Read the model definition and answer for the solid it produces. Units are mm, in the model's axes. A direction names the side the tool comes from. Coordinates: 2 decimals unless noted, no trailing zeros. Order: outer loops, then holes, each group sorted by start corner. A loop starts at its lowest first (then second) coordinate and runs counter-clockwise, first axis right, second up. Notation, with made-up numbers: (-39.5, -5) -> (-25.5, -5) arc R25 cw to (-25.5, 29) -> close; hole circle Ø6 at (33, 88.25). An arc over 180 degrees is marked (long way). Use CSV: the item, a comma, the result in double quotes.
```python
from build123d import *

# Parameters (mm, degrees)
F1_DEPTH    = 8
F3_DEPTH    = 12
F4_R        = 1.5
F5_R        = 1.5
F6_T1_DEPTH = 118.05


# Not quite as in the source:
# - a fillet or chamfer that OpenCascade refuses, or shapes differently, is made with other operations: its cross-section is extruded or revolved along the edge and cut away or added


with BuildPart() as f1:
    # F0 (on Top) → F1 (new body)
    with BuildSketch(Plane.XY):
        Polygon((-127.8, 0), (-132.3, 0), (-132.3, -29), (-129.3, -29), (-129.3, -91.6), (3.75, -91.6), (3.75, -29), (6.75, -29), (6.75, 0), (2.25, 0), (2.25, -20), (-2.25, -20), (-2.25, 0), (-6.75, 0), (-6.75, -29), (-3.75, -29), (-3.75, -84.1), (-121.8, -84.1), (-121.8, -29), (-118.8, -29), (-118.8, 0), (-123.3, 0), (-123.3, -20), (-127.8, -20), align=None)
    extrude(amount=F1_DEPTH)

    # F2 (on face) → F3 (join)
    with BuildSketch(Plane.XY.offset(8)):
        Polygon((-127.8, 0), (-132.3, 0), (-132.3, -29), (-118.8, -29), (-118.8, 0), (-123.3, 0), (-123.3, -20), (-127.8, -20), align=None)
        Polygon((-2.25, 0), (-6.75, 0), (-6.75, -29), (6.75, -29), (6.75, 0), (2.25, 0), (2.25, -20), (-2.25, -20), align=None)
    extrude(amount=F3_DEPTH)

    # F4
    f4_edges = [f1.edges().sort_by_distance(p)[0] for p in [
        (-129.3, -29, 4),
        (-125.55, -29, 8),
        (-121.8, -29, 4),
        (-3.75, -29, 4),
        (0, -29, 8),
        (3.75, -29, 4),
    ]]
    fillet(f4_edges, radius=F4_R)

    # F5
    f5_edges = [f1.edges().sort_by_distance(p)[0] for p in [
        (-132.3, -29, 10),
        (-125.55, -29, 20),
        (-118.8, -29, 10),
        (6.75, -29, 10),
        (0, -29, 20),
        (-6.75, -29, 10),
    ]]
    fillet(f5_edges, radius=F5_R)

    # F6: fillet of radius 5 on 2 edges, made by hand

    # F6_s2 → F6_t1 (cut)
    with BuildSketch(Plane.YZ.offset(-121.8)):
        with BuildLine():
            ThreePointArc((-84.1, 3), (-85.5644660941, 6.5355339059), (-89.1, 8))
            Line((-89.1, 8), (-84.1, 8))
            Line((-84.1, 8), (-84.1, 3))
        make_face()
        with BuildLine():
            ThreePointArc((-89.1, 0), (-85.5644660941, 1.4644660941), (-84.1, 5))
            Line((-84.1, 5), (-84.1, 0))
            Line((-84.1, 0), (-89.1, 0))
        make_face()
    extrude(amount=F6_T1_DEPTH, mode=Mode.SUBTRACT)


solid = f1.part
```
Item 1: Find section B-B, the plane z = 16. Give the vertices of the cut face in (x, y).
Return value:
outline,"(-132.3, -27.5) arc R1.5 ccw to (-130.8, -29) -> (-120.3, -29) arc R1.5 ccw to (-118.8, -27.5) -> (-118.8, 0) -> (-123.3, 0) -> (-123.3, -20) -> (-127.8, -20) -> (-127.8, 0) -> (-132.3, 0) -> close; (-6.75, -27.5) arc R1.5 ccw to (-5.25, -29) -> (5.25, -29) arc R1.5 ccw to (6.75, -27.5) -> (6.75, 0) -> (2.25, 0) -> (2.25, -20) -> (-2.25, -20) -> (-2.25, 0) -> (-6.75, 0) -> close"
Item 2: Straight lines are drawn through the part: line 1 along X through (y, z) = (-19, 14.5); line 2 along Y through (x, z) = (-3.5, 10.5); line 3 along X through (y, z) = (-55.5, 2.75). For each, find the intervals that lie inside material, in ascending order.
Return value:
line 1,"x = -132.3 to -127.8, -123.3 to -118.8, -6.75 to -2.25, 2.25 to 6.75"
line 2,"y = -29 to 0"
line 3,"x = -129.3 to -121.8, -3.75 to 3.75"
Item 3: Find section C-C, the plane y = -42.5. Give the vertices of the cut face in (x, z), then the cut area to 3 significant figures.
Return value:
outline,"(-129.3, 0) -> (-121.8, 0) -> (-121.8, 8) -> (-129.3, 8) -> close; (-3.75, 0) -> (3.75, 0) -> (3.75, 8) -> (-3.75, 8) -> close"
area,"120 mm^2"
Item 4: The mould has two halves that part along X. Classify faces 1 (the flat face through (6.75, -14, 10)), 2 (the flat face through (-118.8, -14, 10)), 3 (the flat face through (5, 0, 10)), 4 (the flat face through (-129.3, -61, 4)): +X half, -X half, draft (parallel to the pull), parting line (faces both ways), or undercut.
Return value:
face 1,"+X half"
face 2,"undercut"
face 3,"draft"
face 4,"-X half"
Item 5: A tool of negligible diameter and unlimited length cuts with its end or side. For faces 5 (the flat face through (-126, -29, 14)), 6 (the flat face through (-6.75, -14, 10)), 7 (the flat face through (3, -14, 20)), from which of +Z, -Z, +X, -X, +Y, -Y can it reach the whole face along a straight path? Write none if from no direction.
Return value:
face 5,"+Z, +X, -X, -Y"
face 6,"+Z, -Z, +Y"
face 7,"+Z, +X, -X, +Y, -Y"
Item 6: Find section D-D, the plane x = -39. Give the vertices of the cut face in (y, z).
Return value:
outline,"(-91.6, 0) -> (-89.1, 0) arc R5 ccw to (-84.2, 4) arc R5 ccw to (-89.1, 8) -> (-91.6, 8) -> close"
Item 7: Each of these flat-tipped pins is pushed along its axis until it touches: P1, Ø2.5, axis at y = -52, z = 4, coming from the +X side; P2, Ø4, axis at y = -68, z = 4.5, coming from the -X side; P3, Ø4.5, axis at x = 1.5, z = 14.5, coming from the -Y side. Where does it stop, or does it pass through?
Return value:
P1,"stops at x = 3.75"
P2,"stops at x = -129.3"
P3,"stops at y = -29"
Item 8: Find section A-A, the plane y = -13. Give the vertices of the cut face in (x, z).
Return value:
outline,"(-132.3, 0) -> (-127.8, 0) -> (-127.8, 20) -> (-132.3, 20) -> close; (-123.3, 0) -> (-118.8, 0) -> (-118.8, 20) -> (-123.3, 20) -> close; (-6.75, 0) -> (-2.25, 0) -> (-2.25, 20) -> (-6.75, 20) -> close; (2.25, 0) -> (6.75, 0) -> (6.75, 20) -> (2.25, 20) -> close"
